Can you work these out from the model? Positions are in its coordinate system, mm. Face numbers are marked on the shaded views. A direction names the side the tool comes from. Give positions to 0.01 mm unless a question says otherwise; leave off trailing zeros. Write each loop counter-clockwise with the first axis right and the second up, starting at its lowest first coordinate (ties: lowest second). Pieces come first, ordered by that corner, then holes.
1. Suppose I cut it at B-B (y = -28). Please give me the cut outline in (x, z).
2. I'm going to push flat-ended pins straight in: pin 1 (19 mm diameter, centred on x = 38, y = -24, fed in from +Z); pin 2 (14.5 mm diameter, centred on x = 45, y = -20, fed in from -Z); pin 3 (3 mm diameter, centred on x = -5.5, y = -11.5, fed in from -Z); pin 4 (12 mm diameter, centred on x = 20.5, z = -10.5, fed in from +Y). Where does each tip first touch, or does it pass through?
3. Suppose I cut it at D-D (y = -3). Please give me the cut outline in (x, z).
4. Suppose I cut it at A-A (z = -88). Please give me the cut outline in (x, y), and give its area (3 significant figures).
5. On a 3-axis mill with a long thin cutter (end or side, diameter ignored), from which of +Z, -Z, +X, -X, +Y, -Y can I reach the whole of each face in a straight line? I mean the marked faces 5, 6 and 7. Say none if no direction works.
6. Thinking about a two-plate mould opening in X: for the marked faces 1, 2, 3 and 4, which applies, pulls with the +X half, pulls with the -X half, needs draft (parallel to the pull), parting line crosses it, or undercut?
7. If I drill on probe 1 along Y at (x, z) = (38, -8); probe 2 along Y at (x, z) = (2.75, -96); probe 3 along X at (y, z) = (-34, -58), over which ranges is the centre line in solid material (lowest first)?
8. Suppose I cut it at C-C (x = 32). Please give me the cut outline in (y, z).
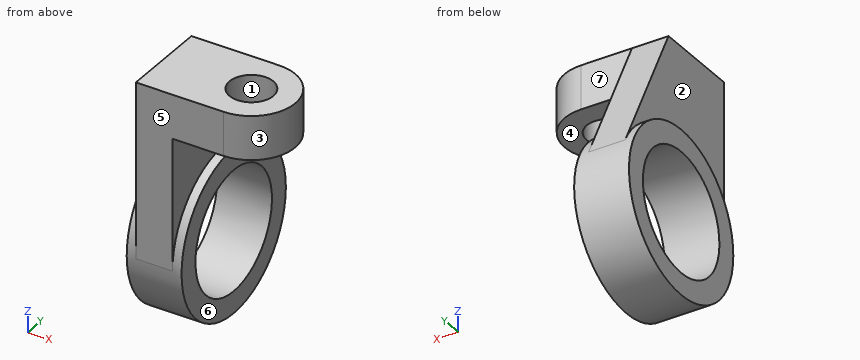
```python
from build123d import *

# Parameters (mm, degrees)
EXTRUDE_1_DEPTH = 10
SKETCH_1_4_R    = 45
SKETCH_1_4_R_2  = 33
EXTRUDE_2_DEPTH = 15
SKETCH_2_R      = 12
EXTRUDE_3_DEPTH = 24


with BuildPart() as part:
    # Sketch 1 → Extrude 1 (new, symmetric)
    with BuildSketch(Plane(origin=(0, 0, 0), x_dir=(0, 0, -1), z_dir=(1, 0, 0))):
        with BuildLine():
            Line((76.168577762, 37.394488387), (0, 0))
            Line((0, 0), (0, -48))
            Line((0, -48), (96, -48))
            ThreePointArc((96, -48), (52.166496961, -13.179587973), (76.168577762, 37.394488387))
        make_face()
    extrude(amount=EXTRUDE_1_DEPTH, both=True)

    # Sketch 1_4 → Extrude 2 (add, symmetric)
    with BuildSketch(Plane(origin=(0, 0, 0), x_dir=(0, 0, -1), z_dir=(1, 0, 0))):
        with Locations((96, -3)):
            Circle(SKETCH_1_4_R)
        with Locations((96, -3)):
            Circle(SKETCH_1_4_R_2, mode=Mode.SUBTRACT)
    extrude(amount=EXTRUDE_2_DEPTH, both=True)

    # Sketch 2 → Extrude 3 (add)
    with BuildSketch(Plane.XY):
        with BuildLine():
            Line((10, -48), (38, -48))
            ThreePointArc((38, -48), (62, -24), (38, 0))
            Line((38, 0), (10, 0))
            Line((10, 0), (10, -48))
        make_face()
        with Locations((38, -24)):
            Circle(SKETCH_2_R, mode=Mode.SUBTRACT)
    extrude(amount=-EXTRUDE_3_DEPTH)


solid = part.part
```
Checks:
1. outline: (-15, -133.42) - (15, -133.42) - (15, -117.54) - (-15, -117.54) - close; (-15, -74.46) - (15, -74.46) - (15, -58.58) - (10, -58.58) - (10, -24) - (26.69, -24) - (26.69, 0) - (-10, 0) - (-10, -58.58) - (-15, -58.58) - close; (49.31, -24) - (61.66, -24) - (61.66, 0) - (49.31, 0) - close
2. pin 1: passes through
2. pin 2: stops at z = -24
2. pin 3: stops at z = -140.45
2. pin 4: stops at y = 0
3. outline: (-15, -141) - (15, -141) - (15, -129) - (-15, -129) - close; (-15, -63) - (15, -63) - (15, -51) - (10, -51) - (10, -24) - (49.62, -24) - (49.62, 0) - (-10, 0) - (-10, -51) - (-15, -51) - close
4. outline: (-15, -47.28) - (-10, -47.28) - (-10, -48) - (10, -48) - (10, -47.28) - (15, -47.28) - (15, -35.02) - (-15, -35.02) - close; (-15, 29.02) - (15, 29.02) - (15, 41.28) - (-15, 41.28) - close
4. area: 750 mm2
5. face 5: +Z, -Z, +X, -X, -Y
5. face 6: -Z, +X, +Y, -Y
5. face 7: +Z, +X, +Y
6. face 1: undercut
6. face 2: pulls with the -X half
6. face 3: pulls with the +X half
6. face 4: needs draft
7. probe 1: y = -48 to -36, -12 to 0
7. probe 2: y = -48 to -36, 30 to 42
7. probe 3: x = -10 to 10
8. outline: (-48, -24) - (-34.39, -24) - (-34.39, 0) - (-48, 0) - close; (-13.61, -24) - (0, -24) - (0, 0) - (-13.61, 0) - close
